Work out the finished part from the listing and answer in its coordinate system (mm). A direction names the side the tool comes from. Round coordinates to 2 decimals unless told otherwise and drop trailing zeros. Write each loop counter-clockwise with the first axis right and the second up, starting at its lowest first coordinate (ties: lowest second). Pieces come first, ordered by that corner, then holes. Notation, with made-up numbers: M -28,70 L -11,70 A9 cw -11,83 Z; hole C -31.75,36 d5. An arc over 180 degrees is marked long. Answer in a Markdown table with one row per item.
```python
from build123d import *

# Parameters (mm, degrees)
SKETCH1_W                   = 153.92
SKETCH1_H                   = 153.92
SKETCH1_R                   = 1.5
SKETCH1_W_2                 = 53
SKETCH1_H_2                 = 52
BOSS_EXTRUDE1_DEPTH         = 25.95
TAP_DRILL_FOR_M4X0_7_TAP2_D = 3.3
SKETCH3_R                   = 55
SKETCH3_W                   = 53
SKETCH3_H                   = 52
BOSS_EXTRUDE3_DEPTH         = 20
SKETCH5_R                   = 3.225
CUT_EXTRUDE1_DEPTH          = 6.35
FILLET2_R                   = 1.5


with BuildPart() as part:
    # Sketch1 → Boss-Extrude1 (new body)
    with BuildSketch(Plane(origin=(0, 0, 0), x_dir=(1, 0, 0), z_dir=(0, 1, 0))):
        Rectangle(SKETCH1_W, SKETCH1_H)
        with Locations(Location((31.5, 0, 0), (0, 0, 270))):
            Circle(SKETCH1_R, mode=Mode.SUBTRACT)
        Rectangle(SKETCH1_W_2, SKETCH1_H_2, mode=Mode.SUBTRACT)
    extrude(amount=-BOSS_EXTRUDE1_DEPTH)

    # Tap Drill for M4x0.7 Tap2 (through all)
    with Locations(Plane(origin=(-60.5282, 0, -60.5282), x_dir=(0, 0, 1), z_dir=(0, 1, 0))):
        with Locations((0, 0), (121.0564, 0), (121.0564, 121.0564), (0, 121.0564)):
            Hole(TAP_DRILL_FOR_M4X0_7_TAP2_D / 2)

    # Sketch3 → Boss-Extrude3 (add)
    with BuildSketch(Plane.XZ.offset(25.95)):
        with Locations(Location((0, 0, 0), (0, 0, 90))):
            Circle(SKETCH3_R)
        Rectangle(SKETCH3_W, SKETCH3_H, mode=Mode.SUBTRACT)
    extrude(amount=BOSS_EXTRUDE3_DEPTH)

    # Sketch5 → Cut-Extrude1 (cut)
    with BuildSketch(Plane.XZ.offset(45.95)):
        with Locations(Location((-37.5, 0, 0), (0, 0, 270))):
            Circle(SKETCH5_R)
        with Locations(Location((37.5, 0, 0), (0, 0, 270))):
            Circle(SKETCH5_R)
    extrude(amount=-CUT_EXTRUDE1_DEPTH, mode=Mode.SUBTRACT)

    # Fillet2
    fillet2_edges = [part.edges().sort_by_distance(p)[0] for p in [
        (-76.96, -12.975, 76.96),
        (-76.96, -12.975, -76.96),
        (76.96, -12.975, -76.96),
        (76.96, -12.975, 76.96),
    ]]
    fillet(fillet2_edges, radius=FILLET2_R)


solid = part.part
```
1. Given pin 1 (5 mm diameter, centred on x = 38, z = 0, fed in from -Y); pin 2 (0.9 mm diameter, centred on x = 31, z = 0, fed in from +Y); pin 3 (6 mm diameter, centred on x = -18.5, y = -37, fed in from +Z), each flat-ended and moving along its own axis, determine where each tip first touches the part or whether it passes through.
Calculated:
| item | result |
|---|---|
| pin 1 | stops at y = -39.6 |
| pin 2 | stops at y = -25.95 |
| pin 3 | stops at z = 52.77 |
2. The part is cut by section B-B (z = 17). Determine the outline of the cut face in (x, y).
Calculated:
| item | result |
|---|---|
| outline | M -76.96,-25.95 L -52.31,-25.95 L -52.31,-45.95 L -26.5,-45.95 L -26.5,0 L -76.96,0 Z; M 26.5,-45.95 L 52.31,-45.95 L 52.31,-25.95 L 76.96,-25.95 L 76.96,0 L 26.5,0 Z |
3. The part is cut by section D-D (y = -9.5). Determine the outline of the cut face in (x, z), plus the area to 3 significant figures.
Calculated:
| item | result |
|---|---|
| outline | M -76.96,-75.46 A1.5 ccw -75.46,-76.96 L 75.46,-76.96 A1.5 ccw 76.96,-75.46 L 76.96,75.46 A1.5 ccw 75.46,76.96 L -75.46,76.96 A1.5 ccw -76.96,75.46 Z; hole C -60.53,-60.53 d3.3; hole C -60.53,60.53 d3.3; hole M -26.5,-26 L 26.5,-26 L 26.5,26 L -26.5,26 Z; hole C 31.5,0 d3; hole C 60.53,-60.53 d3.3; hole C 60.53,60.53 d3.3 |
| area | 20,900 mm² |
4. Consider line 1 along X through (y, z) = (-42.5, 0) (3 decimals); line 2 along X through (y, z) = (-18, 0); line 3 along X through (y, z) = (-25.5, -15.5). Determine where each line is inside the solid, lowest interval first. Write a range as from..to.
Calculated:
| item | result |
|---|---|
| line 1 | x = -55..-40.725, -34.275..-26.5, 26.5..34.275, 40.725..55 |
| line 2 | x = -76.96..-26.5, 26.5..30, 33..76.96 |
| line 3 | x = -76.96..-26.5, 26.5..76.96 |
5. Determine the mould class of faces 1 (the cylindrical face through (40.7, -42.8, 0.4)), 2 (the flat face through (-76.96, -13, 1)), 3 (the flat face through (-18.2, -25.95, -52.4)) for opening direction X: released by +X, released by -X, zero draft, split by the parting line, or undercut.
Calculated:
| item | result |
|---|---|
| face 1 | undercut |
| face 2 | released by -X |
| face 3 | zero draft |
6. The part is cut by section A-A (y = -35). Determine the outline of the cut face in (x, z).
Calculated:
| item | result |
|---|---|
| outline | C 0,0 d110; hole M -26.5,-26 L 26.5,-26 L 26.5,26 L -26.5,26 Z |
7. The part is cut by section C-C (x = -22). Determine the outline of the cut face in (y, z), plus the area to 3 significant figures.
Calculated:
| item | result |
|---|---|
| outline | M -45.95,-50.41 L -25.95,-50.41 L -25.95,-76.96 L 0,-76.96 L 0,-26 L -45.95,-26 Z; M -45.95,26 L 0,26 L 0,76.96 L -25.95,76.96 L -25.95,50.41 L -45.95,50.41 Z |
| area | 3,620 mm² |
8. A tool of negligible diameter and unlimited length cuts with its end or side. For faces 4 (the flat face through (0, -23, 26)), 5 (the flat face through (76.96, -13, 1)), 6 (the cylindrical face through (48.794, -35.81, 25.379)), from which of +Z, -Z, +X, -X, +Y, -Y can it reach the whole face along a straight path? Write none if from no direction.
Calculated:
| item | result |
|---|---|
| face 4 | +Y, -Y |
| face 5 | +Z, -Z, +X, +Y, -Y |
| face 6 | -Y |
